from build123d import *

# Parameters (mm, degrees)
F0_W     = 250
F0_H     = 350
F1_DEPTH = 25
F2_T     = -2.5
F3_W     = 49
F3_H     = 49
F4_DEPTH = 25


with BuildPart() as f1:
    # F0 (on Front) → F1 (new body)
    with BuildSketch(Plane.XZ):
        with Locations((69.741823, 120.105962)):
            Rectangle(F0_W, F0_H)
    extrude(amount=F1_DEPTH)

    # F2
    f2_openings = [f1.faces().sort_by_distance(p)[0] for p in [
        (69.741823, -25, 120.105962),
    ]]
    offset(amount=F2_T, openings=f2_openings)

    # F3 (on face) → F4 (cut)
    with BuildSketch(Plane.XZ):
        with Locations((130.241823, 230.605962)):
            Rectangle(F3_W, F3_H)
    extrude(amount=F4_DEPTH, mode=Mode.SUBTRACT)


solid = f1.part
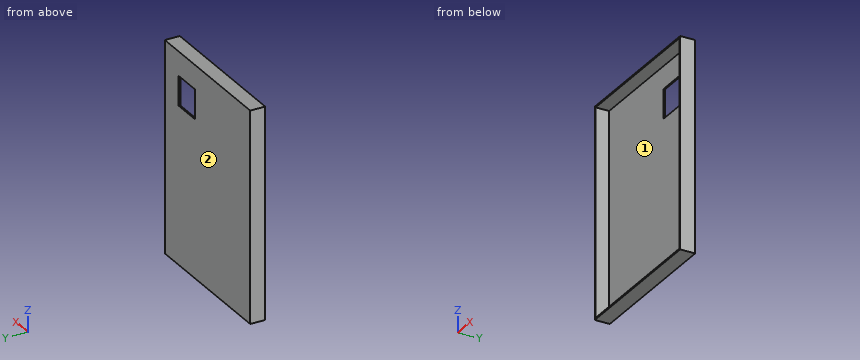
The model under review builds one solid part; all positions refer to its coordinate system, in mm. Face numbers are marked on the shaded views. Give positions to 0.01 mm unless a question says otherwise; leave off trailing zeros. Loops run counter-clockwise (first coordinate to the right, second up) from the corner with the lowest first, then second, coordinate; pieces in that order, holes last. Notation, with made-up numbers: (22, 30.5) -> (44, 30.5) arc R18 ccw to (44, 42.5) -> close; hole circle Ø9 at (21, -17). An arc over 180 degrees is marked (long way). Answer as a JSON object with one key per item and string values. Group by question number.
Q1. Take a section at A-A (z = 235.5). Write out the cut boundary in (x, y), plus the area to 3 significant figures.
Q2. Take a section at D-D (x = 178). Write out the cut boundary in (y, z), plus the area to 4 significant figures.
Q3. Draft analysis for pull direction X (two halves, no side actions). For the marked faces 1 and 2, state which applies: pulls with the +X half, pulls with the -X half, needs draft (parallel to the pull), parting line crosses it, or undercut.
Q4. Wall thickness on line 1 along X through (y, z) = (-19.25, 179); line 2 along Z through (x, y) = (63.5, -19); line 3 along Y through (x, z) = (10.5, 267): over which ranges is each line inside the solid? List them lowest first.
Q5. Take a section at B-B (x = 122.5). Write out the cut boundary in (y, z), plus the area to 3 significant figures.
Q6. Take a section at C-C (y = -13.5). Write out the cut boundary in (x, z), plus the area to 4 significant figures.
Q7. Insertion check: pin 1 (8 mm diameter, centred on x = 112.5, z = 68.5, fed in from +Y); pin 2 (1 mm diameter, centred on x = 49, z = 45.5, fed in from -Y). Each pin has a flat end and moves straight along its axis. Give the tip position at first contact, or say it passes through.
Answer below:
{
 "1": {"outline": "(-55.26, -25) -> (-52.76, -25) -> (-52.76, -2.5) -> (105.74, -2.5) -> (105.74, 0) -> (-55.26, 0) -> close; (154.74, -2.5) -> (192.24, -2.5) -> (192.24, -25) -> (194.74, -25) -> (194.74, 0) -> (154.74, 0) -> close", "area": "615 mm2"},
 "2": {"outline": "(-25, -54.89) -> (0, -54.89) -> (0, 295.11) -> (-25, 295.11) -> (-25, 292.61) -> (-2.5, 292.61) -> (-2.5, -52.39) -> (-25, -52.39) -> close", "area": "987.5 mm2"},
 "3": {"face 1": "undercut", "face 2": "needs draft"},
 "4": {"line 1": "x = -55.26 to -52.76, 192.24 to 194.74", "line 2": "z = -54.89 to -52.39, 292.61 to 295.11", "line 3": "y = -2.5 to 0"},
 "5": {"outline": "(-25, -54.89) -> (0, -54.89) -> (0, 206.11) -> (-2.5, 206.11) -> (-2.5, -52.39) -> (-25, -52.39) -> close; (-25, 292.61) -> (-2.5, 292.61) -> (-2.5, 255.11) -> (0, 255.11) -> (0, 295.11) -> (-25, 295.11) -> close", "area": "865 mm2"},
 "6": {"outline": "(-55.26, -54.89) -> (194.74, -54.89) -> (194.74, 295.11) -> (-55.26, 295.11) -> close; hole (-52.76, -52.39) -> (192.24, -52.39) -> (192.24, 292.61) -> (-52.76, 292.61) -> close", "area": "2,975 mm2"},
 "7": {"pin 1": "stops at y = 0", "pin 2": "stops at y = -2.5"}
}
